```python
from build123d import *

# Parameters (mm, degrees)
F2_R     = 0.5
F3_DEPTH = 52


with BuildPart() as f1:
    # F0 (on Front) → F1 (revolve)
    with BuildSketch(Plane.XZ):
        with BuildLine():
            Line((-9.5, 0), (0, 0))
            ThreePointArc((0, 0), (-2.782486, 6.717514), (-9.5, 9.5))
            Line((-9.5, 9.5), (-42.213703, 9.5))
            ThreePointArc((-42.213703, 9.5), (-47.19787, 8.040891), (-51.638326, 5.347701))
            ThreePointArc((-51.638326, 5.347701), (-53.107777, 4.5324), (-54.764356, 4.25))
            Line((-54.764356, 4.25), (-62, 4.25))
            Line((-62, 4.25), (-64, 3.75))
            Line((-64, 3.75), (-64, 0))
            Line((-64, 0), (-56, 0))
            Line((-56, 0), (-9.5, 0))
        make_face()
    revolve(axis=Axis((-32, 0, 0), (-1, 0, 0)))

    # F2 (on face) → F3 (cut)
    with BuildSketch(Plane(origin=(-64, 0, 0), x_dir=(0, -1, 0), z_dir=(-1, 0, 0))):
        Circle(F2_R)
    extrude(amount=-F3_DEPTH, mode=Mode.SUBTRACT)


solid = f1.part
```
Build history of the part. All positions in model axes, mm. A direction names the side the tool comes from. Give positions to 0.01 mm unless a question says otherwise; leave off trailing zeros. Loops run counter-clockwise (first coordinate to the right, second up) from the corner with the lowest first, then second, coordinate; pieces in that order, holes last.
1) Band-saw the part on B-B on x = -59. List the corners of the cut face in (y, z), then the cut area to 3 significant figures.
Values follow:
outline: circle Ø8.5 at (0, 0); hole circle Ø1 at (0, 0)
area: 56.0 mm2
2) Band-saw the part on A-A on x = -35. List the corners of the cut face in (y, z), then the cut area to 3 significant figures.
Values follow:
outline: circle Ø19 at (0, 0); hole circle Ø1 at (0, 0)
area: 283 mm2
3) Probe line 1 along Z through (x, y) = (-46, 0); line 2 along Y through (x, z) = (-56, 2); line 3 along Z through (x, y) = (-50, 0). List the from-to ranges inside material, lowest first.
Values follow:
line 1: z = -8.52 to -0.5, 0.5 to 8.52
line 2: y = -3.75 to 3.75
line 3: z = -6.53 to -0.5, 0.5 to 6.53
4) Drop flat-ended pins along their axis: P1, Ø8, axis at x = -53, y = -0.5, coming from the -Z side; P2, Ø4, axis at y = 0.5, z = 5, coming from the +X side; P3, Ø3, axis at y = 5.5, z = 3, coming from the +X side. Give the stop position or say it passes through.
Values follow:
P1: stops at z = -7.13
P2: stops at x = -0.49
P3: stops at x = -1.28
5) 3-axis set-ups, long thin cutter, end or side, ignore diameter. For faces 1 (the face through (-58.433, 3.584, 2.285)), 2 (the face through (-26.09, -8.43, 4.38)): which of +Z, -Z, +X, -X, +Y, -Y reach the whole face in a straight line?
Values follow:
face 1: -X
face 2: +X, -X
